from build123d import *

# Parameters (mm, degrees)
SKETCH1_R      = 12.7
EXTRUDE1_DEPTH = 10.000000066


with BuildPart() as part:
    # Sketch1 → Extrude1 (new body)
    with BuildSketch(Plane.XY):
        with BuildLine():
            Line((0, 0), (50.8, 0))
            Line((50.8, 0), (50.8, 38.1))
            Line((50.8, 38.1), (0, 38.1))
            ThreePointArc((0, 38.1), (-19.05, 19.05), (0, 0))
        make_face()
        with Locations((0, 19.05)):
            Circle(SKETCH1_R, mode=Mode.SUBTRACT)
    extrude(amount=-EXTRUDE1_DEPTH)


solid = part.part
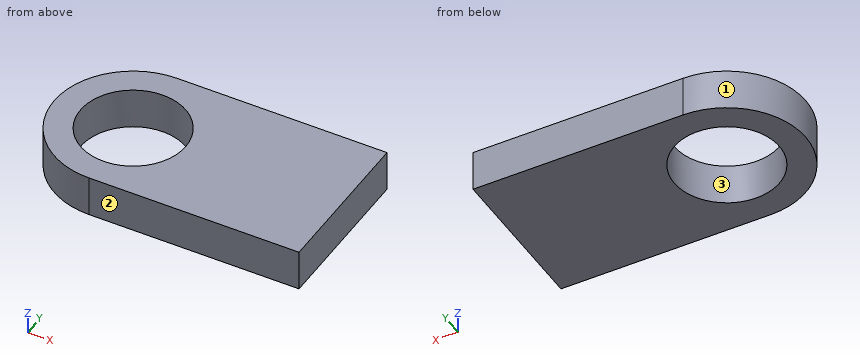
The model under review builds one solid part; all positions refer to its coordinate system, in mm. Face numbers are marked on the shaded views. Give positions to 0.01 mm unless a question says otherwise; leave off trailing zeros. Order: outer loops, then holes, each group sorted by start corner. A loop starts at its lowest first (then second) coordinate and runs counter-clockwise, first axis right, second up. Notation, with made-up numbers: M 37.5,58 L 49.5,58 A21 ccw 49.5,74 Z; hole C -0.5,18.25 d9. An arc over 180 degrees is marked long. Use one line per item in the form item = value. Start each with the question number.
Item 1: We need section B-B on x = -4.5. Give the boundary of the cut face in (y, z), plus the area to 3 significant figures.
Item 2: We need section A-A on y = 19.05. Give the boundary of the cut face in (x, z), plus the area to 4 significant figures.
Item 3: The part is to be moulded in two halves that separate along X. For the marked faces 1, 2 and 3, say which applies: pulls with the +X half, pulls with the -X half, needs draft (parallel to the pull), parting line crosses it, or undercut.
Item 4: To check wall thickness, follow line 1 along Y through (x, z) = (0, -2); line 2 along Y through (x, z) = (3.5, -3.5); line 3 along X through (y, z) = (14, -2). State the ranges of each line that lie inside material, in increasing order. Write a range as from..to.
Item 5: Insertion check: pin 1 Ø1.5 at (x, z) = (-6.5, -7.5) entering from -Y; pin 2 Ø1.5 at (x, z) = (-7, -9) entering from -Y; pin 3 Ø1.5 at (y, z) = (14.5, -6.5) entering from -X. Each pin has a flat end and moves straight along its axis. Give the tip position at first contact, or say it passes through.
Item 6: We need section D-D on y = 35.5. Give the boundary of the cut face in (x, z).
Item 7: We need section C-C on z = -0.75. Give the boundary of the cut face in (x, y), plus the area to 3 significant figures.
Completed:
q1.outline = M 0.54,-10 L 7.17,-10 L 7.17,0 L 0.54,0 Z; M 30.93,-10 L 37.56,-10 L 37.56,0 L 30.93,0 Z
q1.area = 133 mm²
q2.outline = M -19.05,-10 L -12.7,-10 L -12.7,0 L -19.05,0 Z; M 12.7,-10 L 50.8,-10 L 50.8,0 L 12.7,0 Z
q2.area = 444.5 mm²
q3.face_1 = pulls with the -X half
q3.face_2 = needs draft
q3.face_3 = undercut
q4.line_1 = 0..6.35, 31.75..38.1
q4.line_2 = 0..6.84, 31.26..38.1
q4.line_3 = -18.37..-11.65, 11.65..50.8
q5.pin_1 = 0.89
q5.pin_2 = 1.05
q5.pin_3 = -18.67
q6.outline = M -9.61,-10 L 50.8,-10 L 50.8,0 L -9.61,0 Z
q7.outline = M 0,0 L 50.8,0 L 50.8,38.1 L 0,38.1 A19.05 ccw Z; hole C 0,19.05 d25.4
q7.area = 2,000 mm²
